from build123d import *

# Parameters (mm, degrees)
CROQUIS2_W                   = 120
CROQUIS2_H                   = 120
SALIENTE_EXTRUIR1_DEPTH      = 90
VACIADO2_T                   = -4
CROQUIS3_W                   = 136
CROQUIS3_H                   = 136
CROQUIS3_W_2                 = 116
CROQUIS3_H_2                 = 116
CORTAR_EXTRUIR_L_MINA1_DEPTH = 30
REDONDEO3_R                  = 10


with BuildPart() as part:
    # Croquis2 → Saliente-Extruir1 (new body)
    with BuildSketch(Plane(origin=(0, 0, 0), x_dir=(1, 0, 0), z_dir=(0, 1, 0))):
        Rectangle(CROQUIS2_W, CROQUIS2_H)
    extrude(amount=SALIENTE_EXTRUIR1_DEPTH)

    # Vaciado2
    vaciado2_openings = [part.faces().sort_by_distance(p)[0] for p in [
        (0, 90, 0),
    ]]
    offset(amount=VACIADO2_T, openings=vaciado2_openings, kind=Kind.INTERSECTION)

    # Croquis3 → Cortar-Extruir-L_mina1 (cut)
    with BuildSketch(Plane(origin=(0, 90, 0), x_dir=(1, 0, 0), z_dir=(0, 1, 0))):
        Rectangle(CROQUIS3_W, CROQUIS3_H)
        Rectangle(CROQUIS3_W_2, CROQUIS3_H_2, mode=Mode.SUBTRACT)
    extrude(amount=-CORTAR_EXTRUIR_L_MINA1_DEPTH, mode=Mode.SUBTRACT)

    # Redondeo3
    redondeo3_edges = [part.edges().sort_by_distance(p)[0] for p in [
        (56, 47, 56),
        (56, 47, -56),
        (-56, 47, -56),
        (-56, 47, 56),
        (60, 30, 60),
        (-60, 30, 60),
        (-60, 30, -60),
        (60, 30, -60),
        (58, 75, 58),
        (-58, 75, 58),
        (-58, 75, -58),
        (58, 75, -58),
    ]]
    fillet(redondeo3_edges, radius=REDONDEO3_R)


solid = part.part
Source: CAD feature listing. Evaluate the final solid. Frame: model axes, mm. A direction names the side the tool comes from. Give positions to 0.01 mm unless a question says otherwise; leave off trailing zeros. Write each loop counter-clockwise with the first axis right and the second up, starting at its lowest first coordinate (ties: lowest second). Pieces come first, ordered by that corner, then holes. Notation, with made-up numbers: M 60.5,67.5 L 112.5,67.5 A14 cw 112.5,92.5 Z; hole C -35,45.25 d8. An arc over 180 degrees is marked long. Return JSON: item names as keys, results as strings. Group by question number.
1) Cut plane D-D, the plane y = 62. Output: boundary loops of the cut face in (x, z), then the cut area to 3 significant figures.
2) Set-up query: faces 5 (the face through (55.15, 74.79, -54.99)), 6 (the face through (-1, 75, 58)), 7 (the face through (53.15, 46.4, -52.99)). Return all of +Z, -Z, +X, -X, +Y, -Y with unobstructed straight access to the full face (end or side cutting, diameter ignored); none if empty.
3) Ray query, L1, parallel to X at y = 57.5, z = -34; L2, parallel to X at y = 83, z = -40. Return the intervals inside material, ascending.
4) Cut plane C-C, the plane z = 34.5. Output: boundary loops of the cut face in (x, y), then the cut area to 3 significant figures.
5) Draft query along Z for faces 1 (the face through (60, 30, 1)), 2 (the face through (-1, 75, -58)), 3 (the face through (-1, 4, -1)), 4 (the face through (-57.15, 30.42, 56.99)). Return one class per face: released by +Z, released by -Z, zero draft, split by the parting line, or undercut.
6) First-contact query: pin 1 Ø15 at (y, z) = (81, 17.5) entering from -X; pin 2 Ø9 at (x, y) = (-23, 73) entering from +Z; pin 3 Ø15 at (y, z) = (79.5, -13) entering from +X. Flat tips, straight axial feed; report the tip coordinate or a pass-through.
7) Cut plane A-A, the plane x = 41. Output: boundary loops of the cut face in (y, z), then the cut area to 3 significant figures.
8) Cut plane B-B, the plane y = 24.5. Output: boundary loops of the cut face in (x, z), then the cut area to 3 significant figures.
Data:
{
 "1": {"outline": "M -58,-48 A10 ccw -48,-58 L 48,-58 A10 ccw 58,-48 L 58,48 A10 ccw 48,58 L -48,58 A10 ccw -58,48 Z; hole M -56,-46 A10 ccw -46,-56 L 46,-56 A10 ccw 56,-46 L 56,46 A10 ccw 46,56 L -46,56 A10 ccw -56,46 Z", "area": "912 mm²"},
 "2": {"face 5": "-Z, +X, +Y", "face 6": "+Z, +X, -X, +Y", "face 7": "+Y"},
 "3": {"L1": "x = -60 to -56, 56 to 60", "L2": "x = -58 to -56, 56 to 58"},
 "4": {"outline": "M -60,0 L 60,0 L 60,60 L 58,60 L 58,90 L 56,90 L 56,4 L -56,4 L -56,90 L -58,90 L -58,60 L -60,60 Z", "area": "1,050 mm²"},
 "5": {"face 1": "zero draft", "face 2": "released by -Z", "face 3": "undercut", "face 4": "released by +Z"},
 "6": {"pin 1": "stops at x = -58", "pin 2": "stops at z = 58", "pin 3": "stops at x = 58"},
 "7": {"outline": "M 0,-60 L 60,-60 L 60,-58 L 90,-58 L 90,-56 L 4,-56 L 4,56 L 90,56 L 90,58 L 60,58 L 60,60 L 0,60 Z", "area": "1,050 mm²"},
 "8": {"outline": "M -60,-50 A10 ccw -50,-60 L 50,-60 A10 ccw 60,-50 L 60,50 A10 ccw 50,60 L -50,60 A10 ccw -60,50 Z; hole M -56,-46 A10 ccw -46,-56 L 46,-56 A10 ccw 56,-46 L 56,46 A10 ccw 46,56 L -46,56 A10 ccw -56,46 Z", "area": "1,860 mm²"}
}
